CAD build for the part. Positions are in the model's coordinates, mm. Face numbers are marked on the shaded views. A direction names the side the tool comes from. Round coordinates to 2 decimals unless told otherwise and drop trailing zeros. Loops run counter-clockwise (first coordinate to the right, second up) from the corner with the lowest first, then second, coordinate; pieces in that order, holes last.
from build123d import *

# Parameters (mm, degrees)
F1_DEPTH = 20
F2_R     = 20
F3_DEPTH = 11.146497
F4_R     = 5


with BuildPart() as f1:
    # F0 (on Front) → F1 (new body)
    with BuildSketch(Plane.XZ):
        Polygon((26.680096, 11.804356), (14.646225, 25.232092), (-2.982007, 29.022026), (-19.471213, 21.726533), (-28.523077, 6.132242), (-26.680096, -11.804356), (-14.646225, -25.232092), (2.982007, -29.022026), (19.471213, -21.726533), (28.523077, -6.132242), align=None)
    extrude(amount=F1_DEPTH)

    # F2 (on face) → F3 (cut)
    with BuildSketch(Plane.XZ.offset(20)):
        Circle(F2_R)
    extrude(amount=-F3_DEPTH, mode=Mode.SUBTRACT)

    # F4
    f4_edges = [f1.edges().sort_by_distance(p)[0] for p in [
        (-11.22661, 0, 25.374279),
        (-19.471213, -10, 21.726533),
        (-28.523077, -10, 6.132242),
        (-23.997145, 0, 13.929387),
        (-23.997145, -20, 13.929387),
        (-26.680096, -10, -11.804356),
        (-27.601587, 0, -2.836057),
        (-27.601587, -20, -2.836057),
        (-20.66316, 0, -18.518224),
        (-14.646225, -10, -25.232092),
        (2.982007, -10, -29.022026),
        (-5.832109, 0, -27.127059),
        (-5.832109, -20, -27.127059),
        (19.471213, -10, -21.726533),
        (11.22661, 0, -25.374279),
        (11.22661, -20, -25.374279),
        (28.523077, -10, -6.132242),
        (23.997145, 0, -13.929387),
        (23.997145, -20, -13.929387),
        (26.680096, -10, 11.804356),
        (27.601587, 0, 2.836057),
        (27.601587, -20, 2.836057),
        (14.646225, -10, 25.232092),
        (20.66316, 0, 18.518224),
        (20.66316, -20, 18.518224),
        (-2.982007, -10, 29.022026),
        (5.832109, 0, 27.127059),
        (5.832109, -20, 27.127059),
        (-11.22661, -20, 25.374279),
        (-20.66316, -20, -18.518224),
    ]]
    fillet(f4_edges, radius=F4_R)


solid = f1.part
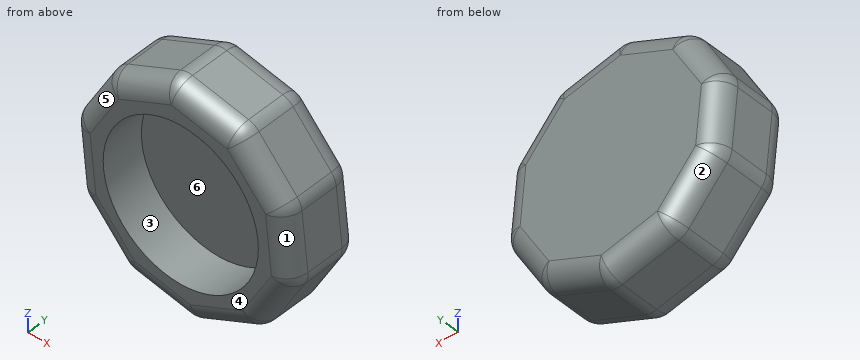
Item 1: Cut at A-A (y = -13.75). List the corners of the cut face in (x, z).
Verdict:
outline: (-28.36, 4.52) - (-26.85, -10.19) arc R5 ccw to (-25.6, -13.01) - (-15.73, -24.02) arc R5 ccw to (-13.06, -25.57) - (1.39, -28.68) arc R5 ccw to (4.47, -28.36) - (17.99, -22.38) arc R5 ccw to (20.29, -20.32) - (27.71, -7.54) arc R5 ccw to (28.36, -4.52) - (26.85, 10.19) arc R5 ccw to (25.6, 13.01) - (15.73, 24.02) arc R5 ccw to (13.06, 25.57) - (-1.39, 28.68) arc R5 ccw to (-4.47, 28.36) - (-17.99, 22.38) arc R5 ccw to (-20.29, 20.32) - (-27.71, 7.54) arc R5 ccw to start; hole circle Ø40 at (0, 0)
Item 2: Wall check: L1, parallel to Z at x = 0, y = -17.5; L2, parallel to Y at x = -6, z = 5; L3, parallel to Y at x = 2, z = -24. Give the ranges that are in metal, low to high.
Verdict:
L1: z = -27.7 to -20, 20 to 27.7
L2: y = -8.85 to 0
L3: y = -19.99 to -0.01
Item 3: Flat gauge pins, fed straight in: P1, Ø8, axis at y = -16.5, z = 17.5, coming from the +X side; P2, Ø4, axis at x = -5.5, y = -16, coming from the +Z side; P3, Ø12, axis at x = 14.5, y = -15, coming from the -Z side; P4, Ø5, axis at x = -4.5, z = -17, coming from the -Y side. Where does each tip first touch, or does it go through?
Verdict:
P1: stops at x = 25.02
P2: stops at z = 28.64
P3: stops at z = -26.58
P4: stops at y = -20
Item 4: Mould opens along Z. For the marked faces 1, 2, 3 and 4 say: released by +Z, released by -Z, zero draft, split by the parting line, or undercut.
Verdict:
face 1: released by +Z
face 2: released by -Z
face 3: undercut
face 4: zero draft
Item 5: 3-axis set-ups, long thin cutter, end or side, ignore diameter. For the marked faces 5 and 6: which of +Z, -Z, +X, -X, +Y, -Y reach the whole face in a straight line?
Verdict:
face 5: +Z, -X, -Y
face 6: -Y
Item 6: Cut at B-B (y = -4). List the corners of the cut face in (x, z), plus the area to 3 significant figures.
Verdict:
outline: (-28.26, 4.53) - (-26.75, -10.18) arc R4.9 ccw to (-25.52, -12.95) - (-15.66, -23.95) arc R4.9 ccw to (-13.04, -25.47) - (1.41, -28.58) arc R4.9 ccw to (4.43, -28.27) - (17.94, -22.29) arc R4.9 ccw to (20.2, -20.27) - (27.62, -7.49) arc R4.9 ccw to (28.26, -4.53) - (26.75, 10.18) arc R4.9 ccw to (25.52, 12.95) - (15.66, 23.95) arc R4.9 ccw to (13.04, 25.47) - (-1.41, 28.58) arc R4.9 ccw to (-4.43, 28.27) - (-17.94, 22.29) arc R4.9 ccw to (-20.2, 20.27) - (-27.62, 7.49) arc R4.9 ccw to start
area: 2,480 mm2
